Autodesk Inventor part; units mm, degrees
ref_plane "ANBAU_XY" through (0, 0, 0) normal (0, 0, -1) x (1, 0, 0)
ref_plane "ANBAU_YZ" through (0, 0, 0) normal (1, 0, 0) x (0, -1, 0)
ref_plane "ANBAU_ZX" through (0, 0, 0) normal (0, -1, 0) x (0, 0, -1)
sketch "Sketch_1" plane through (0, 0, 0) normal (1, 0, 0) x (0, 1, 0)
  line L0 (0, -5.5) -> (0, 13.4)
  line L1 (0, 13.4) -> (3.4785, 13.4)
  line L2 (3.4785, 13.4) -> (5.7347, 13.0022)
  arc A0 (5.9, 12.8052) -> (5.7347, 13.0022) centre (5.7, 12.8052) ccw
  line L3 (5.9, 12.8052) -> (5.9, 11.9)
  line L4 (5.9, 11.9) -> (4.2535, 11.9)
  arc A1 (4.2535, 11.9) -> (3.8785, 11.525) centre (4.2535, 11.525) ccw
  line L5 (3.8785, 11.525) -> (3.8785, 11)
  line L6 (3.8785, 11) -> (4.5136, 11)
  line L7 (4.5136, 11) -> (4.655, 10.8586)
  line L8 (4.655, 10.8586) -> (4.655, 10.6)
  line L9 (4.655, 10.6) -> (4.858, 10.6)
  line L10 (4.858, 10.6) -> (4.9, 10)
  line L11 (4.9, 10) -> (4.9, 0.6)
  line L12 (4.9, 0.6) -> (4.8, 0.5)
  line L13 (4.8, 0.5) -> (4.9, 0.4)
  line L14 (4.9, 0.4) -> (4.9, 0)
  line L15 (4.9, 0) -> (3.5, 0)
  line L16 (3.5, 0) -> (3.5, -4.8865)
  line L17 (3.5, -4.8865) -> (2.8865, -5.5)
  line L18 (2.8865, -5.5) -> (0, -5.5)
  line L19 (0, -5.5) -> (0, 13.4)
revolve "Revolution1" add sketch "Sketch_1" angle 360 about axis through (0, 0, -5.5) along (0, 0, -1)
thread "Thread1"
sketch "Sketch_2" plane through (0, 0, 13.4) normal (0, 0, 1) x (1, 0, 0)
  line L0 (-11.8, -11.8) -> (11.8, -11.8)
  line L1 (11.8, -11.8) -> (11.8, 11.8)
  line L2 (11.8, 11.8) -> (-11.8, 11.8)
  line L3 (-11.8, 11.8) -> (-11.8, -11.8)
  line L4 (-4.9, 1) -> (-4.9, -1)
  arc A0 (-4.9, -1) -> (4.9, -1) centre (0, -1) ccw
  line L5 (4.9, -1) -> (4.9, 1)
  arc A1 (4.9, 1) -> (-4.9, 1) centre (0, 1) ccw
extrude "Extrusion1" cut sketch "Sketch_2" against normal blind 1.5
sketch "Sketch_3" plane through (0, 0, -5.5) normal (0, 0, 1) x (1, 0, 0)
  line L0 (-2, -1.1547) -> (0, -2.3094)
  line L1 (0, -2.3094) -> (2, -1.1547)
  line L2 (2, -1.1547) -> (2, 1.1547)
  line L3 (2, 1.1547) -> (0, 2.3094)
  line L4 (0, 2.3094) -> (-2, 1.1547)
  line L5 (-2, 1.1547) -> (-2, -1.1547)
extrude "Extrusion2" cut sketch "Sketch_3" along normal blind 7.2
sketch "Sketch_4" plane through (0, 0, 0) normal (1, 0, 0) x (0, 1, 0)
  line L0 (0, 1.7) -> (0, 13.4)
  line L1 (0, 13.4) -> (3.4785, 13.4)
  arc A0 (3.4785, 13.4) -> (3.1785, 13.1) centre (3.4785, 13.1) ccw
  line L2 (3.1785, 13.1) -> (3.1785, 1.7)
  line L3 (3.1785, 1.7) -> (0, 1.7)
  line L4 (0, 1.7) -> (0, 13.4)
revolve "Revolution2" cut sketch "Sketch_4" angle 360 about axis through (0, 0, 1.7) along (0, 0, -1)
ref_plane "ANBAU_XY" through (0, 0, 0) normal (0, 0, -1) x (1, 0, 0)
ref_plane "ANBAU_YZ" through (0, 0, 0) normal (1, 0, 0) x (0, -1, 0)
ref_plane "ANBAU_ZX" through (0, 0, 0) normal (0, -1, 0) x (0, 0, -1)
ref_plane "ANBAU_STD_XY" through (0, 0, 0) normal (0, 0, 1) x (1, 0, 0)
ref_plane "ANBAU_STD_YZ" through (0, 0, 0) normal (1, 0, 0) x (0, 1, 0)
ref_plane "ANBAU_STD_ZX" through (0, 0, 0) normal (0, 1, 0) x (0, 0, 1)
ref_plane "CPV_XY" through (0, 0, 0) normal (0, 0, 1) x (1, 0, 0)
ref_plane "CPV_YZ" through (0, 0, 0) normal (1, 0, 0) x (0, 1, 0)
ref_plane "CPV_ZX" through (0, 0, 0) normal (0, 1, 0) x (0, 0, 1)
ref_plane "CPV_ANBAU_XY" through (0, 0, 0) normal (0, 0, 1) x (1, 0, 0)
ref_plane "CPV_ANBAU_YZ" through (0, 0, 0) normal (1, 0, 0) x (0, 1, 0)
ref_plane "CPV_ANBAU_ZX" through (0, 0, 0) normal (0, 1, 0) x (0, 0, 1)
properties part number "183740"
Verification items for the finished model (mm, model axes). A direction names the side the tool comes from. Give positions to 0.01 mm unless a question says otherwise; leave off trailing zeros. Write each loop counter-clockwise with the first axis right and the second up, starting at its lowest first coordinate (ties: lowest second). Pieces come first, ordered by that corner, then holes. Notation, with made-up numbers: (-1, -28.5) - (43, -28.5) arc R27 cw to (43, -8.5) - close; hole circle Ø6 at (3, 71). An arc over 180 degrees is marked (long way). Answer as CSV lines item,"result". Start each with the question number.
1. Sectioned sample at B-B (z = 3.25). Record the boundary of the cut face in (x, y).
2. Draft check along X on faces 6 (the face through (-3.2, 2.1, 0)), 7 (the face through (1.014, 1.724, -1.95)), 8 (the face through (-0.99, 1.74, -1.95)), 9 (the face through (2.62, -2.86, 11.26)). Enter one of: pulls with the +X half, pulls with the -X half, needs draft (parallel to the pull), parting line crosses it, or undercut.
3. Thickness scan on line 1 (X direction, y = 0, z = 10); line 2 (Y direction, x = 0.5, z = 10); line 3 (Y direction, x = 2, z = 5). Record the ranges inside material, lowest first.
4. Depth check by flat-ended pin: pin 1 (1.8 mm diameter, centred on y = 0, z = -1, fed in from +X); pin 2 (1.2 mm diameter, centred on y = -0.5, z = -2.5, fed in from -X); pin 3 (1.5 mm diameter, centred on x = 0.5, y = 4.5, fed in from -Z). Enter the tip coordinate at first touch or a pass-through.
5. Set-up check for faces 1 (the face through (-0.1, -5.9, 12.5)), 2 (the face through (-4, 2, 11.9)), 3 (the face through (0.1, 5.9, 12.5)), 4 (the face through (-1.341, 3.233, -2.477)), 5 (the face through (-1.014, -1.724, -1.95)): record each of +Z, -Z, +X, -X, +Y, -Y from which the full face is reachable in a straight line by a thin tool's end or side.
6. Sectioned sample at A-A (z = -3.5). Record the boundary of the cut face in (x, y), then the cut area to 3 significant figures.
Derived:
1,outline,"circle Ø9.8 at (0, 0); hole circle Ø6.36 at (0, 0)"
2,face 6,"needs draft"
2,face 7,"undercut"
2,face 8,"undercut"
2,face 9,"parting line crosses it"
3,line 1,"-4.9 to -3.18, 3.18 to 4.9"
3,line 2,"-4.87 to -3.14, 3.14 to 4.87"
3,line 3,"-4.47 to -2.47, 2.47 to 4.47"
4,pin 1,"x = 3.5"
4,pin 2,"x = -3.5"
4,pin 3,"z = 0"
5,face 1,"+Z, -Z, -Y"
5,face 2,"none"
5,face 3,"+Z, -Z, +Y"
5,face 4,"-Z"
5,face 5,"+Z, -Z"
6,outline,"circle Ø7 at (0, 0); hole (-2, -1.15) - (0, -2.31) - (2, -1.15) - (2, 1.15) - (0, 2.31) - (-2, 1.15) - close"
6,area,"24.6 mm²"
